from build123d import *

# Parameters (mm, degrees)
SKETCH1_R             = 4.5
SKETCH1_R_2           = 1.325
BOSS_EXTRUDE1_DEPTH   = 8
BOSS_EXTRUDE1_2_DEPTH = 8
BOSS_EXTRUDE1_3_DEPTH = 8
BOSS_EXTRUDE1_4_DEPTH = 8
BOSS_EXTRUDE2_REACH   = 95.306
SKETCH2_W             = 3
SKETCH2_H             = 27.5
CUT_EXTRUDE1_DEPTH    = 63.503999872
SKETCH4_W             = 44
SKETCH4_H             = 44
SKETCH4_W_2           = 36
SKETCH4_H_2           = 36
BOSS_EXTRUDE3_DEPTH   = 2
SKETCH7_W             = 9.5
SKETCH7_H             = 3
BOSS_EXTRUDE5_DEPTH   = 4.3
CUT_EXTRUDE3_START    = -1
SKETCH8_W             = 5.5
SKETCH8_H             = 5.5
CUT_EXTRUDE3_DEPTH    = 1.8
CHAMFER3_SIZE         = 3
SKETCH9_R             = 1.55
CUT_EXTRUDE4_DEPTH    = 5.4
BOSS_EXTRUDE6_DEPTH   = 4
SKETCH11_R            = 1.5
BOSS_EXTRUDE7_DEPTH   = 0.5
FILLET2_R             = 3
CHAMFER4_SIZE         = 1
CHAMFER5_SIZE         = 2


with BuildPart() as part:
    # Sketch1 → Boss-Extrude1 (new body)
    with BuildSketch(Plane(origin=(0, 0, 0), x_dir=(1, 0, 0), z_dir=(0, 1, 0))):
        with Locations(Location((20, -74.5, 0), (0, 0, 270))):
            Circle(SKETCH1_R)
        with Locations(Location((20, -74.5, 0), (0, 0, 270))):
            Circle(SKETCH1_R_2, mode=Mode.SUBTRACT)
    extrude(amount=BOSS_EXTRUDE1_DEPTH)



with BuildPart() as body_2:
    # Sketch1 → Boss-Extrude1 2 (new body)
    with BuildSketch(Plane(origin=(0, 0, 0), x_dir=(1, 0, 0), z_dir=(0, 1, 0))):
        with Locations(Location((-20, -74.5, 0), (0, 0, 270))):
            Circle(SKETCH1_R)
        with Locations(Location((-20, -74.5, 0), (0, 0, 270))):
            Circle(SKETCH1_R_2, mode=Mode.SUBTRACT)
    extrude(amount=BOSS_EXTRUDE1_2_DEPTH)


with BuildPart() as body_3:
    # Sketch1 → Boss-Extrude1 3 (new body)
    with BuildSketch(Plane(origin=(0, 0, 0), x_dir=(1, 0, 0), z_dir=(0, 1, 0))):
        with BuildLine():
            Line((-24.5, -34.5), (-24.5, -25.5))
            Line((-24.5, -25.5), (-15.5, -25.5))
            Line((-15.5, -25.5), (-15.5, -34.5))
            ThreePointArc((-15.5, -34.5), (-20, -39), (-24.5, -34.5))
        make_face()
        with Locations(Location((-20, -34.5, 0), (0, 0, 270))):
            Circle(SKETCH1_R_2, mode=Mode.SUBTRACT)
    extrude(amount=BOSS_EXTRUDE1_3_DEPTH)

    # Boss-Extrude2: up to this face of the body (flat: up to its plane)
    boss_extrude2_end = Plane(body_3.part.faces().sort_by_distance((-24.5, 4, 30))[0])
    # Sketch2 → Boss-Extrude2 (add, up to the picked face)
    with BuildSketch(Plane(origin=(24.5, 0, 0), x_dir=(0, 0, -1), z_dir=(1, 0, 0)), mode=Mode.PRIVATE) as boss_extrude2_sk1:
        with Locations((-27, 13.75)):
            Rectangle(SKETCH2_W, SKETCH2_H)
    boss_extrude2_tool1 = split(extrude(boss_extrude2_sk1.sketch, amount=-BOSS_EXTRUDE2_REACH, mode=Mode.PRIVATE), bisect_by=boss_extrude2_end, keep=Keep.BOTH, mode=Mode.PRIVATE)


with BuildPart() as body_4:
    # Sketch1 → Boss-Extrude1 4 (new body)
    with BuildSketch(Plane(origin=(0, 0, 0), x_dir=(1, 0, 0), z_dir=(0, 1, 0))):
        with BuildLine():
            Line((24.5, -34.5), (24.5, -25.5))
            Line((24.5, -25.5), (15.5, -25.5))
            Line((15.5, -25.5), (15.5, -34.5))
            ThreePointArc((15.5, -34.5), (20, -39), (24.5, -34.5))
        make_face()
        with Locations(Location((20, -34.5, 0), (0, 0, 270))):
            Circle(SKETCH1_R_2, mode=Mode.SUBTRACT)
    extrude(amount=BOSS_EXTRUDE1_4_DEPTH)


with BuildPart() as body_3_1:
    add(body_3.part)

    add(body_4.part)  # Boss-Extrude2 merges body 4
    add(boss_extrude2_tool1.solids().sort_by(Axis((24.5, 13.75, 27), (-1, 0, 0)))[0])

    # Sketch3 → Cut-Extrude1 (cut, through all)
    with BuildSketch(Plane.XY.offset(28.5)):
        Polygon((-24.5, 8), (-9, 27.5), (-24.5, 27.5), align=None)
        Polygon((9, 27.5), (24.5, 8), (24.5, 27.5), align=None)
        Polygon((-15.5, 8), (-15.5, 0), (15.5, 0), (15.5, 8), (6.358974359, 19.5), (-6.358974359, 19.5), align=None)
    extrude(amount=-CUT_EXTRUDE1_DEPTH, mode=Mode.SUBTRACT)


with BuildPart() as part_1:
    add(part.part)

    add(body_2.part)  # Boss-Extrude3 merges body 2

    add(body_3_1.part)  # Boss-Extrude3 merges body 3
    # Sketch4 → Boss-Extrude3 (add)
    with BuildSketch(Plane.XZ):
        with Locations((0, 54.5)):
            Rectangle(SKETCH4_W, SKETCH4_H)
        with Locations((0, 54.5)):
            Rectangle(SKETCH4_W_2, SKETCH4_H_2, mode=Mode.SUBTRACT)
    extrude(amount=-BOSS_EXTRUDE3_DEPTH)

    # Sketch7 → Boss-Extrude5 (add)
    with BuildSketch(Plane(origin=(0, 27.5, 0), x_dir=(1, 0, 0), z_dir=(0, 1, 0))):
        with Locations((0, -30)):
            Rectangle(SKETCH7_W, SKETCH7_H)
    extrude(amount=-BOSS_EXTRUDE5_DEPTH)

    # Sketch8 → Cut-Extrude3 (cut)
    with BuildSketch(Plane(origin=(0, 27.5, 0), x_dir=(1, 0, 0), z_dir=(0, 1, 0)).offset(CUT_EXTRUDE3_START)):
        with Locations((0, -28.75)):
            Rectangle(SKETCH8_W, SKETCH8_H)
    extrude(amount=-CUT_EXTRUDE3_DEPTH, mode=Mode.SUBTRACT)

    # Chamfer3
    chamfer3_edges = [part_1.edges().sort_by_distance(p)[0] for p in [
        (0, 23.2, 28.5),
    ]]
    chamfer(chamfer3_edges, length=CHAMFER3_SIZE - 0.0001)  # a hair under: the kernel refuses the full size

    # Sketch9 → Cut-Extrude4 (cut)
    with BuildSketch(Plane(origin=(0, 27.5, 0), x_dir=(1, 0, 0), z_dir=(0, 1, 0))):
        with Locations(Location((0, -28.75, 0), (0, 0, 270))):
            Circle(SKETCH9_R)
    extrude(amount=-CUT_EXTRUDE4_DEPTH, mode=Mode.SUBTRACT)

    # Sketch10 → Boss-Extrude6 (add)
    with BuildSketch(Plane.XZ):
        with BuildLine():
            Line((-24.5, 25.5), (-27.25, 25.5))
            ThreePointArc((-27.25, 25.5), (-33.226647927, 30.971152617), (-28.303578206, 37.406773482))
            Line((-28.303578206, 37.406773482), (-22, 38.531128874))
            Line((-22, 38.531128874), (-22, 25.5))
            Line((-22, 25.5), (-24.5, 25.5))
        make_face()
        Polygon((-27.25, 28.324573519), (-24.5, 29.91228676), (-24.5, 33.08771324), (-27.25, 34.675426481), (-30, 33.08771324), (-30, 29.91228676), align=None, mode=Mode.SUBTRACT)
    boss_extrude6 = extrude(amount=-BOSS_EXTRUDE6_DEPTH)

    # Sketch11 → Boss-Extrude7 (add)
    with BuildSketch(Plane.XZ):
        Polygon((-30, 33.08771324), (-30, 29.91228676), (-27.25, 28.324573519), (-24.5, 29.91228676), (-24.5, 33.08771324), (-27.25, 34.675426481), align=None)
        with Locations(Location((-27.25, 31.5, 0), (0, 0, 270))):
            Circle(SKETCH11_R, mode=Mode.SUBTRACT)
    boss_extrude7 = extrude(amount=-BOSS_EXTRUDE7_DEPTH)

    # Mirror1: Boss-Extrude6, Boss-Extrude7 across plane
    add(boss_extrude6.mirror(Plane(origin=(0, 0, 0), x_dir=(0, 0, 1), z_dir=(1, 0, 0))))
    add(boss_extrude7.mirror(Plane(origin=(0, 0, 0), x_dir=(0, 0, 1), z_dir=(1, 0, 0))))

    # Fillet2
    fillet2_edges = [part_1.edges().sort_by_distance(p)[0] for p in [
        (15.968871126, 1, 76.5),
        (-18, 1, 70.468871126),
        (-15.968871126, 1, 76.5),
        (-22, 1, 70.468871126),
        (-15.968871126, 1, 72.5),
        (15.968871126, 1, 36.5),
        (-15.968871126, 1, 36.5),
        (15.5, 1, 32.5),
        (-15.5, 1, 32.5),
        (18, 1, 70.468871126),
        (-18, 1, 38.531128874),
        (22, 1, 70.468871126),
        (18, 1, 38.531128874),
        (15.968871126, 1, 72.5),
    ]]
    fillet(fillet2_edges, radius=FILLET2_R)

    # Chamfer4
    chamfer4_edges = [part_1.edges().sort_by_distance(p)[0] for p in [
        (15.5, 4, 25.5),
        (-15.5, 4, 25.5),
    ]]
    chamfer(chamfer4_edges, length=CHAMFER4_SIZE)

    # Chamfer5
    chamfer5_edges = [part_1.edges().sort_by_distance(p)[0] for p in [
        (20, 8, 70),
        (-20, 8, 70),
        (-24.5, 8, 31.5),
        (-20, 8, 39),
        (-15.5, 8, 31.5),
        (15.5, 8, 31.5),
        (20, 8, 39),
        (24.5, 8, 31.5),
    ]]
    chamfer(chamfer5_edges, length=CHAMFER5_SIZE)


solid = part_1.part
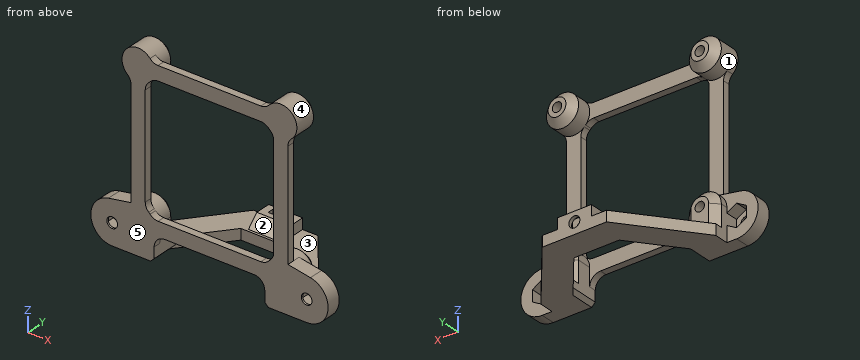
The listing builds one solid part. Answer for the finished solid, in the listing's coordinates (mm). Face numbers are marked on the shaded views. A direction names the side the tool comes from. Round coordinates to 2 decimals unless told otherwise and drop trailing zeros. Order: outer loops, then holes, each group sorted by start corner. A loop starts at its lowest first (then second) coordinate and runs counter-clockwise, first axis right, second up. Notation, with made-up numbers: (-39.75, 85) - (-16.75, 85) arc R22 ccw to (-16.75, 94) - close; hole circle Ø3 at (31.25, -21). An arc over 180 degrees is marked (long way). Write item = value, one per line. Start each with the question number.
1) For a pull along Z with two mould halves and no side action, classify the marked faces 3, 4 and 5 as released by +Z, released by -Z, zero draft, split by the parting line, or undercut.
2) Straight lines are drawn through the part: L1, parallel to X at y = 5.5, z = 74.5 (3 decimals); L2, parallel to Z at x = 20, y = 5.35 (3 decimals); L3, parallel to X at y = 22.8, z = 28.75. For each, find the intervals that lie inside material, in ascending order.
3) Section D-D, the plane y = 25.5 is taken. Write down the section's boundary in (x, z).
4) Section C-C, the plane y = 8.75 is taken. Write down the section's boundary in (x, z), plus the area to 3 significant figures.
5) Given pin 1 (1.4 mm diameter, centred on x = 1, y = 25, fed in from +Z); pin 2 (3 mm diameter, centred on x = 20, z = 34.5, fed in from +Y); pin 3 (8 mm diameter, centred on y = 3.5, z = 28.5, fed in from +X); pin 4 (3.5 mm diameter, centred on x = 27.25, z = 31.5, fed in from +Y), each flat-ended and moving along its own axis, determine where each tip first touches the part or whether it passes through.
6) Section B-B, the plane x = 0 is taken. Count the separate pieces of the cut face and the enclosed holes in it, plus the area to 3 significant figures.
7) Section A-A, the plane z = 54.5 is taken. Write down the section's boundary in (x, y).
8) For the marked faces 1 and 2, determine the directions among +Z, -Z, +X, -X, +Y, -Y from which every point of the face is accessible in a straight line to the end or side of a thin tool.
Results list:
q1.face_3 = released by +Z
q1.face_4 = undercut
q1.face_5 = zero draft
q2.L1 = -24.5 to -21.325, -18.675 to -15.5, 15.5 to 18.675, 21.325 to 24.5
q2.L2 = 25.5 to 33.175, 35.825 to 39, 70 to 73.175, 75.825 to 79
q2.L3 = -4.75 to -1.55, 1.55 to 4.75
q3.outline = (-10.59, 25.5) - (10.59, 25.5) - (10.59, 28.5) - (4.75, 28.5) - (4.75, 31.5) - (2.75, 31.5) - (2.75, 26) - (-2.75, 26) - (-2.75, 31.5) - (-4.75, 31.5) - (-4.75, 28.5) - (-10.59, 28.5) - close
q4.outline = (-23.9, 25.5) - (-14.9, 25.5) - (-14.9, 28.5) - (-23.9, 28.5) - close; (14.9, 25.5) - (23.9, 25.5) - (23.9, 28.5) - (14.9, 28.5) - close
q4.area = 54.0 mm^2
q5.pin_1 = 31.5
q5.pin_2 = 8
q5.pin_3 = 33.25
q5.pin_4 = 0.5
q6.separate_pieces = 4
q6.enclosed_holes = 0
q6.area = 36.3 mm^2
q7.outline = (-22, 0) - (-18, 0) - (-18, 2) - (-22, 2) - close; (18, 0) - (22, 0) - (22, 2) - (18, 2) - close
q8.face_1 = +Y
q8.face_2 = +Z, +X, -X, -Y
